Read the model definition and answer for the solid it produces. Units are mm, in the model's axes. Face numbers are marked on the shaded views. A direction names the side the tool comes from. Give positions to 0.01 mm unless a question says otherwise; leave off trailing zeros. Write each loop counter-clockwise with the first axis right and the second up, starting at its lowest first coordinate (ties: lowest second). Pieces come first, ordered by that corner, then holes. Notation, with made-up numbers: (45, 81) -> (63, 81) arc R10 cw to (63, 95) -> close; hole circle Ø5 at (37.25, 14). An arc over 180 degrees is marked (long way). Use a Markdown table: item, result.
from build123d import *

# Parameters (mm, degrees)
ESBO_O1_R                = 2.05
RESSALTO_EXTRUS_O1_DEPTH = 10
CORTE_EXTRUS_O1_REACH    = 31.766
ESBO_O2_R                = 2
FILETE1_R                = 2


with BuildPart() as part:
    # Esboço1 → Ressalto-extrusão1 (new body)
    with BuildSketch(Plane.XY):
        with BuildLine():
            Line((-7.992042116, -8.75), (-7.992042116, -4.5))
            Line((-7.992042116, -4.5), (-17.992042116, -4.5))
            Line((-17.992042116, -4.5), (-17.992042116, -0.5))
            Line((-17.992042116, -0.5), (-8, -0.5))
            Line((-8, -0.5), (-3.968626967, -0.5))
            ThreePointArc((-3.968626967, -0.5), (4, 0), (-3.968626967, 0.5))
            Line((-3.968626967, 0.5), (-8, 0.5))
            Line((-8, 0.5), (-17.992042116, 0.5))
            Line((-17.992042116, 0.5), (-17.992042116, 4.5))
            Line((-17.992042116, 4.5), (-7.992042116, 4.5))
            Line((-7.992042116, 4.5), (-7.992042116, 8.75))
            ThreePointArc((-7.992042116, 8.75), (0.005510323, 17.001506438), (7.999953669, 8.74698773))
            Line((7.999953669, 8.74698773), (8.000049012, -9.25301227))
            ThreePointArc((8.000049012, -9.25301227), (-0.247502701, -16.997552144), (-7.992042116, -8.75))
        make_face()
        with Locations((0, 12)):
            Circle(ESBO_O1_R, mode=Mode.SUBTRACT)
        with Locations((0, -12)):
            Circle(ESBO_O1_R, mode=Mode.SUBTRACT)
    extrude(amount=RESSALTO_EXTRUS_O1_DEPTH)

    # Corte-extrusão1: up to this face of the body (flat: up to its plane)
    corte_extrus_o1_end = Plane(part.part.faces().sort_by_distance((-12.992042116, 4.5, 5))[0])
    # Esboço2 → Corte-extrusão1 (cut, up to the picked face)
    with BuildSketch(Plane.XZ.offset(4.5), mode=Mode.PRIVATE) as corte_extrus_o1_sk1:
        with Locations((-12.992042116, 5)):
            Circle(ESBO_O2_R)
    corte_extrus_o1_tool1 = split(extrude(corte_extrus_o1_sk1.sketch, amount=-CORTE_EXTRUS_O1_REACH, mode=Mode.PRIVATE), bisect_by=corte_extrus_o1_end, keep=Keep.BOTH, mode=Mode.PRIVATE)
    add(corte_extrus_o1_tool1.solids().sort_by(Axis((-12.992042, -4.5, 5), (0, 1, 0)))[0], mode=Mode.SUBTRACT)

    # Filete1
    filete1_edges = [part.edges().sort_by_distance(p)[0] for p in [
        (-7.992042116, -4.5, 5),
        (-7.992042116, 4.5, 5),
        (-17.992042116, -4.5, 5),
        (-17.992042116, 0.5, 5),
        (-17.992042116, -0.5, 5),
        (-17.992042116, 4.5, 5),
    ]]
    fillet(filete1_edges, radius=FILETE1_R - 0.0001)  # a hair under: the kernel refuses the full size


solid = part.part
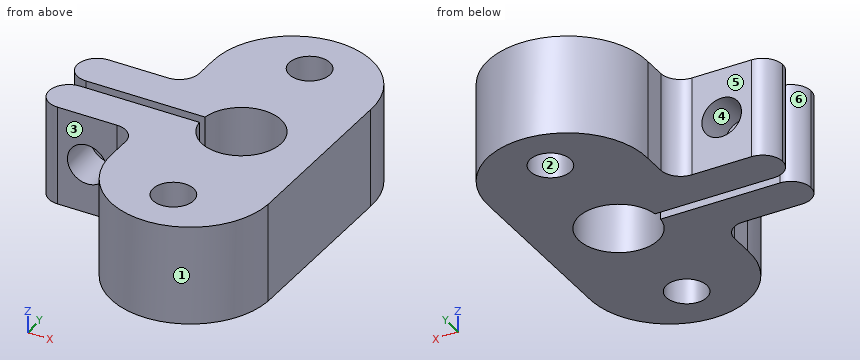
Item 1: A cutting plane is placed at A-A (z = 5). Count the separate pieces of the cut face and the enclosed holes in it, then the cut area to 3 significant figures.
Return value:
| item | result |
|---|---|
| separate pieces | 3 |
| enclosed holes | 2 |
| area | 455 mm^2 |
Item 2: A cutting plane is placed at C-C (y = 2). Give the vertices of the cut face in (x, z).
Return value:
| item | result |
|---|---|
| outline | (-17.93, 0) -> (-3.46, 0) -> (-3.46, 10) -> (-17.93, 10) -> close; (3.46, 0) -> (8, 0) -> (8, 10) -> (3.46, 10) -> close; hole circle Ø4 at (-12.99, 5) |
Item 3: Straight lines are drawn through the part: line 1 along Y through (x, z) = (0, 8.25); line 2 along Y through (x, z) = (-11.25, 6.5); line 3 along Y through (x, z) = (-9, 6). For each, find the intervals that lie inside material, in ascending order. Write a range as [from, to].
Return value:
| item | result |
|---|---|
| line 1 | [-17, -14.05], [-9.95, -4], [4, 9.95], [14.05, 17] |
| line 2 | [-4.5, -0.5], [0.5, 4.5] |
| line 3 | [-4.76, -0.5], [0.5, 4.76] |
Item 4: Each of these flat-tipped pins is pushed along its axis until it touches: P1, Ø1.8, axis at x = -12.5, z = 3, coming from the -Y side; P2, Ø3, axis at y = -4.5, z = 4, coming from the -X side; P3, Ø3, axis at x = -3, z = 6, coming from the -Y side. Where does it stop, or does it pass through?
Return value:
| item | result |
|---|---|
| P1 | y = -4.5 |
| P2 | x = -17.93 |
| P3 | y = -16.86 |
Item 5: For a pull along X with two mould halves and no side action, classify the marked faces 1, 2 and 3 as +X half, -X half, draft (parallel to the pull), parting line (faces both ways), or undercut.
Return value:
| item | result |
|---|---|
| face 1 | parting line |
| face 2 | undercut |
| face 3 | draft |
Item 6: A tool of negligible diameter and unlimited length cuts with its end or side. For the marked faces 4, 5 and 6, from which of +Z, -Z, +X, -X, +Y, -Y can it reach the whole face along a straight path? Write none if from no direction.
Return value:
| item | result |
|---|---|
| face 4 | +Y, -Y |
| face 5 | +Z, -Z, -X, +Y |
| face 6 | +Z, -Z, -X |
Item 7: A cutting plane is placed at B-B (x = 0). Give the vertices of the cut face in (y, z).
Return value:
| item | result |
|---|---|
| outline | (-17, 0) -> (-14.05, 0) -> (-14.05, 10) -> (-17, 10) -> close; (-9.95, 0) -> (-4, 0) -> (-4, 10) -> (-9.95, 10) -> close; (4, 0) -> (9.95, 0) -> (9.95, 10) -> (4, 10) -> close; (14.05, 0) -> (17, 0) -> (17, 10) -> (14.05, 10) -> close |
